Autodesk Inventor part; units mm, degrees
ref_plane "YZ Plane" through (0, 0, 0) normal (1, 0, 0) x (0, 1, 0)
ref_plane "XZ Plane" through (0, 0, 0) normal (0, 1, 0) x (-1, 0, 0)
ref_plane "XY Plane" through (0, 0, 0) normal (0, 0, 1) x (1, 0, 0)
sketch "Sketch1" plane through (0, 0, 0) normal (0, 0, 1) x (1, 0, 0)
  line L0 (0, 0) -> (25.4, 0)
  line L1 (25.4, 25.4) -> (25.4, 76.2)
  line L2 (25.4, 76.2) -> (0, 76.2)
  line L3 (0, 76.2) -> (0, 0)
  line L4 (0, 0) -> (76.2, 0)
  line L5 (76.2, 0) -> (76.2, 25.4)
  line L6 (76.2, 25.4) -> (25.4, 25.4)
  line L7 (0, 25.4) -> (0, 0)
  line L8 (12.7, 76.2) -> (12.7, 63.5) construction
  line L9 (12.7, 63.5) -> (12.7, 38.1) construction
  line L10 (12.7, 38.1) -> (12.7, 12.7) construction
  line L11 (12.7, 12.7) -> (38.1, 12.7) construction
  line L12 (38.1, 12.7) -> (63.5, 12.7) construction
  circle A0 centre (12.7, 63.5) radius 2.5797
  circle A1 centre (12.7, 38.1) radius 2.5797
  circle A2 centre (12.7, 12.7) radius 2.5797
  circle A3 centre (38.1, 12.7) radius 2.5797
  circle A4 centre (63.5, 12.7) radius 2.5797
  dimension "d0" = 25.4
  dimension "d1" = 76.2
  dimension "d2" = 76.2
  dimension "d3" = 25.4
  dimension "d4" = 12.7
  dimension "d5" = 25.4
  dimension "d6" = 25.4
  dimension "d7" = 25.4
  dimension "d8" = 25.4
  dimension "d9" = 5.1594
extrude "Extrusion1" add sketch "Sketch1" along normal blind 3.175
properties part number "L-Guesset"
Verification items for the finished model (mm, model axes). A direction names the side the tool comes from. Round coordinates to 2 decimals unless told otherwise and drop trailing zeros. Write each loop counter-clockwise with the first axis right and the second up, starting at its lowest first coordinate (ties: lowest second). Pieces come first, ordered by that corner, then holes. Notation, with made-up numbers: (5, 33.25) - (11, 33.25) arc R6 cw to (11, 44.25) - close; hole circle Ø1 at (60.5, 49.25). An arc over 180 degrees is marked (long way). Answer as a JSON object with one key per item and string values. Group by question number.
Q1. Section check B-B, the plane y = 12.7. Enter the section's corners in (x, z) (3 decimals).
Q2. Section check C-C, the plane z = 2.1. Enter the section's corners in (x, y).
Q3. Tool access check on faces 5 (the cylindrical face through (14.087, 10.525, 1.565)), 6 (the flat face through (25.4, 50, 2)). Record the directions out of +Z, -Z, +X, -X, +Y, -Y that give a thin tool (end or side, any length) a straight path to the whole face; none if there is none.
Q4. Thickness scan on line 1 (Y direction, x = 12.7, z = 1); line 2 (Y direction, x = 38, z = 1.7); line 3 (Y direction, x = 12, z = 0.6). Record the ranges inside material, lowest first.
Q5. Mould release check, pull along Y, two halves, no side actions. Record for faces 1 (the flat face through (38, 0, 2)), 2 (the flat face through (0, 39, 2)), 3 (the flat face through (13, 76.2, 2)), 4 (the cylindrical face through (40.561, 11.925, 1.565)): released by +Y, released by -Y, zero draft, split by the parting line, or undercut.
Q6. Go/stop test with flat-tipped pins: pin 1 Ø4 at (x, y) = (12.7, 12.7) entering from +Z; pin 2 Ø1.6 at (y, z) = (39, 1) entering from +X. Record where each tip stops, or that it passes through.
Q7. Section check A-A, the plane y = 38.1. Enter the section's corners in (x, z) (3 decimals), plus the area to 3 significant figures.
Found:
{
 "1": {"outline": "(0, 0) - (10.12, 0) - (10.12, 3.175) - (0, 3.175) - close; (15.28, 0) - (35.52, 0) - (35.52, 3.175) - (15.28, 3.175) - close; (40.68, 0) - (60.92, 0) - (60.92, 3.175) - (40.68, 3.175) - close; (66.08, 0) - (76.2, 0) - (76.2, 3.175) - (66.08, 3.175) - close"},
 "2": {"outline": "(0, 0) - (76.2, 0) - (76.2, 25.4) - (25.4, 25.4) - (25.4, 76.2) - (0, 76.2) - close; hole circle Ø5.16 at (12.7, 12.7); hole circle Ø5.16 at (12.7, 38.1); hole circle Ø5.16 at (12.7, 63.5); hole circle Ø5.16 at (38.1, 12.7); hole circle Ø5.16 at (63.5, 12.7)"},
 "3": {"face 5": "+Z, -Z", "face 6": "+Z, -Z, +X, +Y"},
 "4": {"line 1": "y = 0 to 10.12, 15.28 to 35.52, 40.68 to 60.92, 66.08 to 76.2", "line 2": "y = 0 to 10.12, 15.28 to 25.4", "line 3": "y = 0 to 10.22, 15.18 to 35.62, 40.58 to 61.02, 65.98 to 76.2"},
 "5": {"face 1": "released by -Y", "face 2": "zero draft", "face 3": "released by +Y", "face 4": "undercut"},
 "6": {"pin 1": "passes through", "pin 2": "stops at x = 25.4"},
 "7": {"outline": "(0, 0) - (10.12, 0) - (10.12, 3.175) - (0, 3.175) - close; (15.28, 0) - (25.4, 0) - (25.4, 3.175) - (15.28, 3.175) - close", "area": "64.3 mm^2"}
}
